Model file for the job. Use its own axes, mm. Face numbers are marked on the shaded views. A direction names the side the tool comes from. Round coordinates to 2 decimals unless told otherwise and drop trailing zeros. Loops run counter-clockwise (first coordinate to the right, second up) from the corner with the lowest first, then second, coordinate; pieces in that order, holes last. Notation, with made-up numbers: (-7.75, -30.75) - (12.25, -30.75) arc R24 cw to (12.25, 2.25) - close; hole circle Ø11 at (-29.5, -29.75). An arc over 180 degrees is marked (long way). Answer as a JSON object with one key per item and string values.
from build123d import *

# Parameters (mm, degrees)
F0_W     = 25.4
F0_H     = 7.62
F1_DEPTH = 12.7
F3_DEPTH = 2.54
F5_DEPTH = 2.54


with BuildPart() as f1:
    # F0 (on Top) → F1 (new body)
    with BuildSketch(Plane.XY):
        with Locations((12.7, -3.81)):
            Rectangle(F0_W, F0_H)
    extrude(amount=F1_DEPTH)

    # F2 (on face) → F3 (join)
    with BuildSketch(Plane.YZ.offset(25.4)):
        with BuildLine():
            Line((-5.715, 6.35), (-3.81, 6.35))
            Line((-3.81, 6.35), (-1.905, 6.35))
            ThreePointArc((-1.905, 6.35), (-3.81, 8.255), (-5.715, 6.35))
        make_face()
        with BuildLine():
            Line((-1.905, 6.35), (-3.81, 6.35))
            Line((-3.81, 6.35), (-5.715, 6.35))
            ThreePointArc((-5.715, 6.35), (-3.81, 4.445), (-1.905, 6.35))
        make_face()
    extrude(amount=F3_DEPTH)

    # F4 (on face) → F5 (join)
    with BuildSketch(Plane(origin=(0, 0, 0), x_dir=(0, -1, 0), z_dir=(-1, 0, 0))):
        with BuildLine():
            Line((1.905, 6.35), (3.81, 6.35))
            Line((3.81, 6.35), (5.715, 6.35))
            ThreePointArc((5.715, 6.35), (3.81, 8.255), (1.905, 6.35))
        make_face()
        with BuildLine():
            Line((5.715, 6.35), (3.81, 6.35))
            Line((3.81, 6.35), (1.905, 6.35))
            ThreePointArc((1.905, 6.35), (3.81, 4.445), (5.715, 6.35))
        make_face()
    extrude(amount=F5_DEPTH)


solid = f1.part
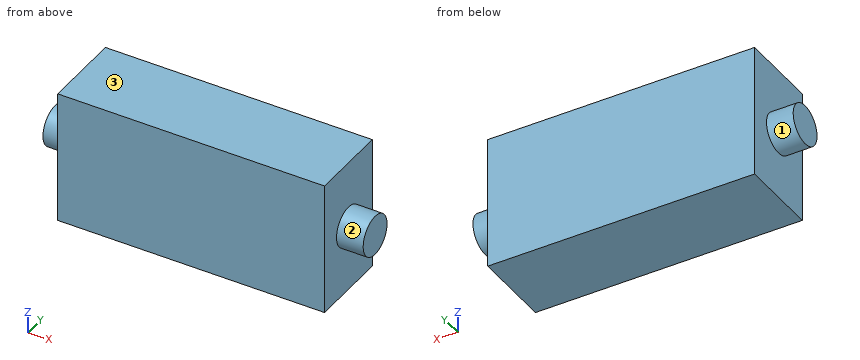
1) Probe probe 1 along X at (y, z) = (-2.25, 4.5); probe 2 along Y at (x, z) = (-1, 6.5). List the from-to ranges inside material, lowest first.
Values follow:
{"probe 1": "0 to 25.4", "probe 2": "-5.71 to -1.91"}
2) Slice it at B-B on z = 6.35. List the corners of the cut face in (x, y) (3 decimals), then the cut area to 3 significant figures.
Values follow:
{"outline": "(-2.54, -5.715) - (0, -5.715) - (0, -7.62) - (25.4, -7.62) - (25.4, -5.715) - (27.94, -5.715) - (27.94, -1.905) - (25.4, -1.905) - (25.4, 0) - (0, 0) - (0, -1.905) - (-2.54, -1.905) - close", "area": "213 mm²"}
3) Tool access for the marked faces 1, 2 and 3: list every direction of +Z, -Z, +X, -X, +Y, -Y with a clear straight run to the whole face (end or side of a thin tool).
Values follow:
{"face 1": "-X", "face 2": "+X", "face 3": "+Z, +X, -X, +Y, -Y"}
4) Slice it at A-A on y = -3.81. List the corners of the cut face in (x, z) (3 decimals), then the cut area to 3 significant figures.
Values follow:
{"outline": "(-2.54, 4.445) - (0, 4.445) - (0, 0) - (25.4, 0) - (25.4, 4.445) - (27.94, 4.445) - (27.94, 8.255) - (25.4, 8.255) - (25.4, 12.7) - (0, 12.7) - (0, 8.255) - (-2.54, 8.255) - close", "area": "342 mm²"}
5) Drop a flat-ended pin along its axis: P1, Ø2.5, axis at y = -5.5, z = 8.5, coming from the -X side. Give the stop position or say it passes through.
Values follow:
{"P1": "x = -2.54"}
6) Slice it at C-C on z = 9. List the corners of the cut face in (x, y), then the cut area to 3 significant figures.
Values follow:
{"outline": "(0, -7.62) - (25.4, -7.62) - (25.4, 0) - (0, 0) - close", "area": "194 mm²"}
7) Slice it at D-D on y = -6. List the corners of the cut face in (x, z).
Values follow:
{"outline": "(0, 0) - (25.4, 0) - (25.4, 12.7) - (0, 12.7) - close"}
